Read the model definition and answer for the solid it produces. Units are mm, in the model's axes. A direction names the side the tool comes from. Round coordinates to 2 decimals unless told otherwise and drop trailing zeros. Write each loop counter-clockwise with the first axis right and the second up, starting at its lowest first coordinate (ties: lowest second). Pieces come first, ordered by that corner, then holes. Notation, with made-up numbers: (62.25, 56.5) - (67.25, 56.5) arc R8 ccw to (67.25, 63.5) - close; hole circle Ø1 at (0.25, -23.5). An arc over 180 degrees is marked (long way). Use one line per item in the form item = value. Start each with the question number.
1) The part is cut by section A-A, the plane y = -34. Give the vertices of the cut face in (x, z).
2) The part is cut by section C-C, the plane z = -2.75. Count the separate pieces of the cut face and the enclosed holes in it, plus the area to 3 significant figures.
3) For faces 4 (the face through (89, -26.35, -3)), 5 (the face through (20, 37.1, -3)), 6 (the face through (-131.1, 5, -3)), determine the directions among +Z, -Z, +X, -X, +Y, -Y from which every point of the face is accessible in a straight line to the end or side of a thin tool.
4) Each of these flat-tipped pins is pushed along its axis until it touches: pin 1 (3 mm diameter, centred on x = -63, z = -4, fed in from +Y); pin 2 (0.9 mm diameter, centred on y = 39, z = -4, fed in from +X); pin 3 (2 mm diameter, centred on x = 101.5, z = -2.5, fed in from +Y). Where does it stop, or does it pass through?
5) For a pull along Y with two mould halves and no side action, classify faces 1 (the face through (131.1, 5, -3)), 2 (the face through (0, 0, -3)), 3 (the face through (-84, 1, -3)) as released by +Y, released by -Y, zero draft, split by the parting line, or undercut.
6) Consider line 1 along Y through (x, z) = (-110, -1.05); line 2 along X through (y, z) = (-27, -4.2); line 3 along X through (y, z) = (-49.5, -4.7). Determine where each line is inside the solid, lowest interval first. Write a range as from..to.
7) The part is cut by section B-B, the plane y = -21. Give the vertices of the cut face in (x, z), plus the area to 3 significant figures.
8) The part is cut by section D-D, the plane y = -5. Give the vertices of the cut face in (x, z), plus the area to 3 significant figures.
from build123d import *

# Parameters (mm, degrees)
BOSS_EXTRUDE1_DEPTH     = 6
CUT_EXTRUDE1_DEPTH      = 150.053681605
CUT_EXTRUDE1_DEPTH_BACK = 150.053681605
SKETCH2_W               = 10
SKETCH2_H               = 5
SKETCH2_W_2             = 5
SKETCH2_H_2             = 10
FILLET1_R               = 10
CUT_EXTRUDE2_DEPTH      = 150.053681605
CUT_EXTRUDE2_DEPTH_BACK = 150.053681605
SKETCH3_W               = 10
SKETCH3_H               = 2.9
SKETCH3_W_2             = 2.9
SKETCH3_H_2             = 10
SKETCH4_W               = 2.9
SKETCH4_H               = 10
CUT_EXTRUDE3_DEPTH      = 150.053681605


with BuildPart() as part:
    # Sketch1 → Boss-Extrude1 (new body)
    with BuildSketch(Plane.XY):
        Polygon((134, -65), (16.25, -65), (16.25, 0), (-16.25, 0), (-16.25, -65), (-134, -65), (-134, 7.5), (-69, 7.5), (-69, 40), (69, 40), (69, 7.5), (134, 7.5), align=None)
    extrude(amount=-BOSS_EXTRUDE1_DEPTH)

    # Sketch2 → Cut-Extrude1 (cut, two sides: drawn at the far end of the back side and taken through both)
    with BuildSketch(Plane.XY.offset(-CUT_EXTRUDE1_DEPTH_BACK)):
        with Locations((-114, 1.15)):
            Rectangle(SKETCH2_W, SKETCH2_H)
        with Locations((-114, -28.85)):
            Rectangle(SKETCH2_W, SKETCH2_H)
        with Locations((-89, -28.85)):
            Rectangle(SKETCH2_W, SKETCH2_H)
        with Locations((-89, 1.15)):
            Rectangle(SKETCH2_W, SKETCH2_H)
        with Locations((-52.6, -20)):
            Rectangle(SKETCH2_W_2, SKETCH2_H_2)
        with Locations((-22.6, -20)):
            Rectangle(SKETCH2_W_2, SKETCH2_H_2)
        with Locations((-52.6, -45)):
            Rectangle(SKETCH2_W_2, SKETCH2_H_2)
        with Locations((-22.6, -45)):
            Rectangle(SKETCH2_W_2, SKETCH2_H_2)
        with Locations((89, -28.85)):
            Rectangle(SKETCH2_W, SKETCH2_H)
        with Locations((114, -28.85)):
            Rectangle(SKETCH2_W, SKETCH2_H)
        with Locations((114, 1.15)):
            Rectangle(SKETCH2_W, SKETCH2_H)
        with Locations((89, 1.15)):
            Rectangle(SKETCH2_W, SKETCH2_H)
    extrude(amount=CUT_EXTRUDE1_DEPTH + CUT_EXTRUDE1_DEPTH_BACK, mode=Mode.SUBTRACT)

    # Fillet1
    fillet1_edges = [part.edges().sort_by_distance(p)[0] for p in [
        (16.25, 0, -3),
        (-16.25, 0, -3),
        (-69, 7.5, -3),
        (69, 7.5, -3),
    ]]
    fillet(fillet1_edges, radius=FILLET1_R)

    # Sketch3 → Cut-Extrude2 (cut, two sides: drawn at the far end of the back side and taken through both)
    with BuildSketch(Plane(origin=(0, 0, -6), x_dir=(-1, 0, 0), z_dir=(0, 0, -1)).offset(-CUT_EXTRUDE2_DEPTH_BACK)):
        with Locations((0, 38.55)):
            Rectangle(SKETCH3_W, SKETCH3_H)
        with Locations((20, 38.55)):
            Rectangle(SKETCH3_W, SKETCH3_H)
        with Locations((40, 38.55)):
            Rectangle(SKETCH3_W, SKETCH3_H)
        with Locations((60, 38.55)):
            Rectangle(SKETCH3_W, SKETCH3_H)
        with Locations((-20, 38.55)):
            Rectangle(SKETCH3_W, SKETCH3_H)
        with Locations((-40, 38.55)):
            Rectangle(SKETCH3_W, SKETCH3_H)
        with Locations((-60, 38.55)):
            Rectangle(SKETCH3_W, SKETCH3_H)
        with Locations((-132.55, -12.5)):
            Rectangle(SKETCH3_W_2, SKETCH3_H_2)
        with Locations((-132.55, 7.5)):
            Rectangle(SKETCH3_W_2, SKETCH3_H_2)
        with Locations((-132.55, -32.5)):
            Rectangle(SKETCH3_W_2, SKETCH3_H_2)
        with Locations((-132.55, -52.5)):
            Rectangle(SKETCH3_W_2, SKETCH3_H_2)
        with Locations((132.55, -52.5)):
            Rectangle(SKETCH3_W_2, SKETCH3_H_2)
        with Locations((132.55, -32.5)):
            Rectangle(SKETCH3_W_2, SKETCH3_H_2)
        with Locations((132.55, -12.5)):
            Rectangle(SKETCH3_W_2, SKETCH3_H_2)
        with Locations((132.55, 7.5)):
            Rectangle(SKETCH3_W_2, SKETCH3_H_2)
    extrude(amount=CUT_EXTRUDE2_DEPTH + CUT_EXTRUDE2_DEPTH_BACK, mode=Mode.SUBTRACT)

    # Sketch4 → Cut-Extrude3 (cut, through all)
    with BuildSketch(Plane(origin=(0, 0, -6), x_dir=(-1, 0, 0), z_dir=(0, 0, -1))):
        with Locations((63.55, 27.1)):
            Rectangle(SKETCH4_W, SKETCH4_H)
        with Locations((63.55, 7.1)):
            Rectangle(SKETCH4_W, SKETCH4_H)
        with Locations((-63.55, 7.1)):
            Rectangle(SKETCH4_W, SKETCH4_H)
        with Locations((-63.55, 27.1)):
            Rectangle(SKETCH4_W, SKETCH4_H)
    extrude(amount=-CUT_EXTRUDE3_DEPTH, mode=Mode.SUBTRACT)


solid = part.part
Geometry results:
q1.outline = (-131.1, -6) - (-16.25, -6) - (-16.25, 0) - (-131.1, 0) - close; (16.25, -6) - (131.1, -6) - (131.1, 0) - (16.25, 0) - close
q2.separate_pieces = 1
q2.enclosed_holes = 16
q2.area = 20,800 mm2
q3.face_4 = +Z, -Z
q3.face_5 = +Z, -Z, +Y
q3.face_6 = +Z, -Z, -X, +Y
q4.pin_1 = 37.1
q4.pin_2 = 69
q4.pin_3 = 7.5
q5.face_1 = zero draft
q5.face_2 = released by -Y
q5.face_3 = undercut
q6.line_1 = -65..-31.35, -26.35..-1.35, 3.65..7.5
q6.line_2 = -134..-119, -109..-94, -84..-16.25, 16.25..84, 94..109, 119..134
q6.line_3 = -131.1..-55.1, -50.1..-25.1, -20.1..-16.25, 16.25..131.1
q7.outline = (-134, -6) - (-55.1, -6) - (-55.1, 0) - (-134, 0) - close; (-50.1, -6) - (-25.1, -6) - (-25.1, 0) - (-50.1, 0) - close; (-20.1, -6) - (-16.25, -6) - (-16.25, 0) - (-20.1, 0) - close; (16.25, -6) - (134, -6) - (134, 0) - (16.25, 0) - close
q7.area = 1,350 mm2
q8.outline = (-134, -6) - (-14.91, -6) - (-14.91, 0) - (-134, 0) - close; (14.91, -6) - (134, -6) - (134, 0) - (14.91, 0) - close
q8.area = 1,430 mm2
